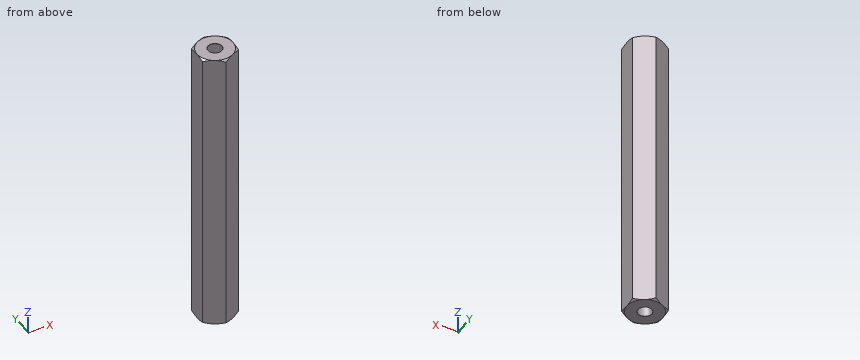
```python
from build123d import *

# Parameters (mm, degrees)
EXTRUDE1_DEPTH          = 50.8
EXTRUDE1_DEPTH_BACK     = 50.8
SKETCH1_R               = 2.413
SKETCH8_OUTSIDE_W       = 392.404
SKETCH8_OUTSIDE_H       = 394.368
SKETCH8_OUTSIDE_R       = 6.35
EXTRUDE4_DEPTH          = 103.061970554
EXTRUDE4_DRAFT          = -60
MIRROR1_COPY_1_SKETCH_W = 392.404
MIRROR1_COPY_1_SKETCH_H = 394.368
MIRROR1_COPY_1_SKETCH_R = 6.35
MIRROR1_COPY_1_DEPTH    = 103.061970554
MIRROR1_COPY_1_DRAFT    = -60


with BuildPart() as part:
    # Sketch1 → Extrude1 (new, two sides: drawn at the far end of the back side and taken through both)
    with BuildSketch(Plane.XY.offset(-EXTRUDE1_DEPTH_BACK)):
        Polygon((0, 7.332348419), (-6.35, 3.666174209), (-6.35, -3.666174209), (0, -7.332348419), (6.35, -3.666174209), (6.35, 3.666174209), align=None)
        Circle(SKETCH1_R, mode=Mode.SUBTRACT)
    extrude(amount=EXTRUDE1_DEPTH + EXTRUDE1_DEPTH_BACK)

    # Extrude3 cone 1 section (through the dimple's axis) → Extrude3 (revolve, cut)
    with BuildSketch(Plane(origin=(0, 0, -50.8), x_dir=(0, 1, 0), z_dir=(1, 0, 0))):
        Polygon((0, 0), (2.4638, 0), (0, 2.642102028), align=None)
    extrude3 = revolve(axis=Axis((0, 0, -50.8), (0, 0, 1)), mode=Mode.SUBTRACT)


with BuildPart() as extrude4_tool:
    # Sketch8 outside → Extrude4 (with draft: the straight prism first)
    with BuildSketch(Plane(origin=(0, 0, -50.8), x_dir=(-1, 0, 0), z_dir=(0, 0, -1))):
        Rectangle(SKETCH8_OUTSIDE_W, SKETCH8_OUTSIDE_H)
        Circle(SKETCH8_OUTSIDE_R, mode=Mode.SUBTRACT)
    extrude(amount=-EXTRUDE4_DEPTH)
    # Extrude4: the draft: its side faces are tilted about the plane it starts from
    extrude4_sides = [extrude4_tool.faces().sort_by_distance(p)[0] for p in [
        (0, -197.184, 0.730985277),
        (-196.202, 0, 0.730985277),
        (0, 197.184, 0.730985277),
        (196.202, 0, 0.730985277),
        (6.35, 0, 0.730985277),
    ]]
    draft(extrude4_sides, Plane(origin=(0, 0, -50.8), x_dir=(-1, 0, 0), z_dir=(0, 0, -1)), EXTRUDE4_DRAFT)


with BuildPart() as part_1:
    add(part.part)

    # Extrude4: cut by extrude4_tool
    add(extrude4_tool.part, mode=Mode.SUBTRACT)

    # Mirror1: Extrude3 across plane
    add(extrude3.mirror(Plane.XY), mode=Mode.SUBTRACT)


with BuildPart() as mirror1_copy_1_tool:
    # Mirror1 copy 1 sketch → Mirror1 copy 1 (with draft: the straight prism first)
    with BuildSketch(Plane(origin=(0, 0, 50.8), x_dir=(-1, 0, 0), z_dir=(0, 0, 1))):
        Rectangle(MIRROR1_COPY_1_SKETCH_W, MIRROR1_COPY_1_SKETCH_H)
        Circle(MIRROR1_COPY_1_SKETCH_R, mode=Mode.SUBTRACT)
    extrude(amount=-MIRROR1_COPY_1_DEPTH)
    # Mirror1 copy 1: the draft: its side faces are tilted about the plane it starts from
    mirror1_copy_1_sides = [mirror1_copy_1_tool.faces().sort_by_distance(p)[0] for p in [
        (0, -197.184, -0.730985277),
        (-196.202, 0, -0.730985277),
        (0, 197.184, -0.730985277),
        (196.202, 0, -0.730985277),
        (6.35, 0, -0.730985277),
    ]]
    draft(mirror1_copy_1_sides, Plane(origin=(0, 0, 50.8), x_dir=(-1, 0, 0), z_dir=(0, 0, 1)), MIRROR1_COPY_1_DRAFT)


with BuildPart() as part_2:
    add(part_1.part)

    # Mirror1 copy 1: cut by mirror1_copy_1_tool
    add(mirror1_copy_1_tool.part, mode=Mode.SUBTRACT)


solid = part_2.part
```
Work out the finished part from the listing and answer in its coordinate system (mm). Give positions to 0.01 mm unless a question says otherwise; leave off trailing zeros. Write each loop counter-clockwise with the first axis right and the second up, starting at its lowest first coordinate (ties: lowest second). Pieces come first, ordered by that corner, then holes.
(1) Straight lines are drawn through the part: line 1 (X direction, y = 0, z = 1); line 2 (Y direction, x = 0, z = -21); line 3 (Y direction, x = 2, z = -12.5). For each, find the intervals that lie inside material, in ascending order.
Final values:
line 1: x = -6.35 to -2.41, 2.41 to 6.35
line 2: y = -7.33 to -2.41, 2.41 to 7.33
line 3: y = -6.18 to -1.35, 1.35 to 6.18
(2) The part is cut by section A-A on z = -1. Write down the section's boundary in (x, y).
Final values:
outline: (-6.35, -3.67) - (0, -7.33) - (6.35, -3.67) - (6.35, 3.67) - (0, 7.33) - (-6.35, 3.67) - close; hole circle Ø4.83 at (0, 0)
(3) Flat-ended cylindrical pins translate along their axes: pin 1 Ø1 at (x, z) = (-3, 14) entering from -Y; pin 2 Ø4 at (x, z) = (-0.5, -29.5) entering from -Y. Find the tip coordinate at first contact, or state that the pin passes through.
Final values:
pin 1: stops at y = -5.89
pin 2: stops at y = -7.33
